Model file for the job. Use its own axes, mm. Give positions to 0.01 mm unless a question says otherwise; leave off trailing zeros. Write each loop counter-clockwise with the first axis right and the second up, starting at its lowest first coordinate (ties: lowest second). Pieces come first, ordered by that corner, then holes. Notation, with made-up numbers: (20.5, 47.5) - (27.5, 47.5) arc R17 cw to (27.5, 51.5) - close; hole circle Ø11 at (-37.5, -23.5). An arc over 180 degrees is marked (long way). Use CSV: the item, a comma, the result in double quotes.
from build123d import *

# Parameters (mm, degrees)
SKETCH_1_W          = 40
SKETCH_1_H          = 15
EXTRUDE_1_DEPTH     = 2
SKETCH_3_R          = 1.5
CUT_EXTRUDE_1_DEPTH = 2
CUT_EXTRUDE_2_DEPTH = 10
FILLET_1_R          = 5


with BuildPart() as part:
    # 草图1 → 凸台-拉伸1 (new body)
    with BuildSketch(Plane.XY):
        Rectangle(SKETCH_1_W, SKETCH_1_H)
    extrude(amount=EXTRUDE_1_DEPTH)

    # 草图3 → 切除-拉伸1 (cut)
    with BuildSketch(Plane.XY.offset(2)):
        with Locations((-9.982459034, 0.236161147)):
            Circle(SKETCH_3_R)
        with Locations((-17.5, -2.5)):
            Circle(SKETCH_3_R)
    extrude(amount=-CUT_EXTRUDE_1_DEPTH, mode=Mode.SUBTRACT)

    # 草图6 → 切除-拉伸2 (cut)
    with BuildSketch(Plane.XY.offset(2)):
        Polygon((-5, 7.5), (-5, -7.5), (36.148851336, -18.495224014), (30.781609857, 18.543577541), align=None)
    extrude(amount=-CUT_EXTRUDE_2_DEPTH, mode=Mode.SUBTRACT)

    # 圆角1
    fillet_1_edges = [part.edges().sort_by_distance(p)[0] for p in [
        (-5, 7.5, 1),
        (-5, -7.5, 1),
        (-20, -7.5, 1),
        (-20, 7.5, 1),
    ]]
    fillet(fillet_1_edges, radius=FILLET_1_R)


solid = part.part
(1) Saw through at B-B, the plane z = 0.2. List the corners of the cut face in (x, y).
Checked values:
outline,"(-20, -2.5) arc R5 ccw to (-15, -7.5) - (-10, -7.5) arc R5 ccw to (-5, -2.5) - (-5, 2.5) arc R5 ccw to (-10, 7.5) - (-15, 7.5) arc R5 ccw to (-20, 2.5) - close; hole circle Ø3 at (-17.5, -2.5); hole circle Ø3 at (-9.98, 0.24)"
(2) Pull direction Y, two halves, no side cores. Call faces 1 (the face through (-19, -2.43, 1.01)), 2 (the face through (-13, 7.5, 1)), 3 (the face through (-13, 0, 2)): released by +Y, released by -Y, zero draft, split by the parting line, or undercut.
Checked values:
face 1,"undercut"
face 2,"released by +Y"
face 3,"zero draft"
(3) Wall check: probe 1 along Y at (x, z) = (-10, 1.85); probe 2 along X at (y, z) = (-1.5, 1.45); probe 3 along Y at (x, z) = (-17.5, 0.8). Give the ranges that are in metal, low to high. Write a range as [from, to].
Checked values:
probe 1,"y = [-7.5, -1.26], [1.74, 7.5]"
probe 2,"x = [-20, -18.62], [-16.38, -5]"
probe 3,"y = [-6.83, -4], [-1, 6.83]"
(4) Flat gauge pin, fed straight in: P1, Ø1, axis at x = -7, z = 1.5, coming from the -Y side. Where does the tip first touch, or does it go through?
Checked values:
P1,"stops at y = -6.83"
(5) Saw through at D-D, the plane x = -8.25. List the corners of the cut face in (y, z), then the cut area to 3 significant figures.
Checked values:
outline,"(-7.18, 0) - (7.18, 0) - (7.18, 2) - (-7.18, 2) - close"
area,"28.7 mm^2"
(6) Saw through at A-A, the plane x = -17.5. List the corners of the cut face in (y, z), then the cut area to 3 significant figures.
Checked values:
outline,"(-6.83, 0) - (-4, 0) - (-4, 2) - (-6.83, 2) - close; (-1, 0) - (6.83, 0) - (6.83, 2) - (-1, 2) - close"
area,"21.3 mm^2"
(7) Saw through at C-C, the plane y = 5.75. List the corners of the cut face in (x, z), then the cut area to 3 significant figures.
Checked values:
outline,"(-18.8, 0) - (-6.2, 0) - (-6.2, 2) - (-18.8, 2) - close"
area,"25.2 mm^2"
